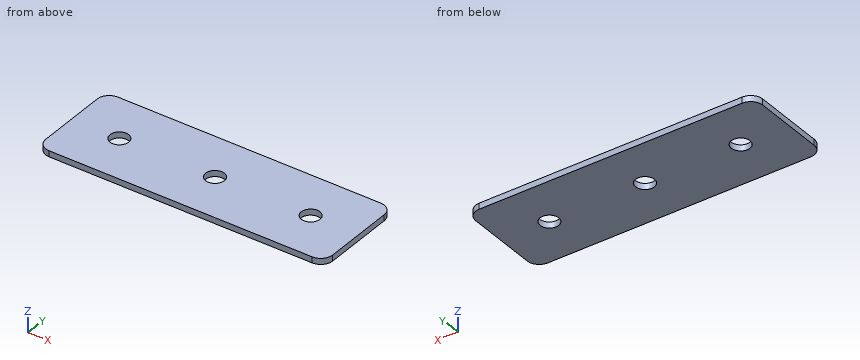
from build123d import *

# Parameters (mm, degrees)
SKETCH1_W           = 76.2
SKETCH1_H           = 25.4
BOSS_EXTRUDE1_DEPTH = 1.5875
SKETCH2_R           = 2.4892
CUT_EXTRUDE1_DEPTH  = 81.337538898
FILLET1_R           = 3.175


with BuildPart() as part:
    # Sketch1 → Boss-Extrude1 (new body)
    with BuildSketch(Plane.XY):
        with Locations((38.1, 12.7)):
            Rectangle(SKETCH1_W, SKETCH1_H)
    extrude(amount=-BOSS_EXTRUDE1_DEPTH)

    # Sketch2 → Cut-Extrude1 (cut, through all)
    with BuildSketch(Plane.XY):
        with Locations((12.7, 12.7)):
            Circle(SKETCH2_R)
        with Locations((38.1, 12.7)):
            Circle(SKETCH2_R)
        with Locations((63.5, 12.7)):
            Circle(SKETCH2_R)
        with Locations((88.9, 12.7)):
            Circle(SKETCH2_R)
        with Locations((114.3, 12.7)):
            Circle(SKETCH2_R)
    extrude(amount=-CUT_EXTRUDE1_DEPTH, mode=Mode.SUBTRACT)

    # Fillet1
    fillet1_edges = [part.edges().sort_by_distance(p)[0] for p in [
        (0, 25.4, -0.79375),
        (76.2, 25.4, -0.79375),
        (76.2, 0, -0.79375),
        (0, 0, -0.79375),
    ]]
    fillet(fillet1_edges, radius=FILLET1_R)


solid = part.part
Can you work these out from the model? Positions are in its coordinate system, mm. Round coordinates to 2 decimals unless told otherwise and drop trailing zeros. Write each loop counter-clockwise with the first axis right and the second up, starting at its lowest first coordinate (ties: lowest second). Pieces come first, ordered by that corner, then holes. Notation, with made-up numbers: (-8, 33.5) -> (35, 33.5) arc R21 cw to (35, 46.5) -> close; hole circle Ø10 at (84, 1.25). An arc over 180 degrees is marked (long way). One line per question, with ' | ' between items. Start each with the question number.
1) Suppose I cut it at C-C on x = 14.5. Write out the boundary of the cut face in (y, z).
2) I'm going to push a flat-ended pin straight in: P1, Ø6.5, axis at x = 12.7, y = 12.7, coming from the -Z side. Where does the tip first touch, or does it pass through?
3) Suppose I cut it at B-B on x = 63.5. Write out the boundary of the cut face in (y, z), then the cut area to 3 significant figures.
4) Suppose I cut it at A-A on y = 12.7. Write out the boundary of the cut face in (x, z).
5) I need wall thicknesses on line 1 (Y direction, x = 63.5, z = -0.4); line 2 (X direction, y = 11.25, z = -1.45); line 3 (X direction, y = 13.5, z = -0.65). Which ranges of each line are inside material? Lowest first, please. Write a range as [from, to].
Return value:
1) outline: (0, -1.59) -> (10.98, -1.59) -> (10.98, 0) -> (0, 0) -> close; (14.42, -1.59) -> (25.4, -1.59) -> (25.4, 0) -> (14.42, 0) -> close
2) P1: stops at z = -1.59
3) outline: (0, -1.59) -> (10.21, -1.59) -> (10.21, 0) -> (0, 0) -> close; (15.19, -1.59) -> (25.4, -1.59) -> (25.4, 0) -> (15.19, 0) -> close | area: 32.4 mm2
4) outline: (0, -1.59) -> (10.21, -1.59) -> (10.21, 0) -> (0, 0) -> close; (15.19, -1.59) -> (35.61, -1.59) -> (35.61, 0) -> (15.19, 0) -> close; (40.59, -1.59) -> (61.01, -1.59) -> (61.01, 0) -> (40.59, 0) -> close; (65.99, -1.59) -> (76.2, -1.59) -> (76.2, 0) -> (65.99, 0) -> close
5) line 1: y = [0, 10.21], [15.19, 25.4] | line 2: x = [0, 10.68], [14.72, 36.08], [40.12, 61.48], [65.52, 76.2] | line 3: x = [0, 10.34], [15.06, 35.74], [40.46, 61.14], [65.86, 76.2]
